Model file for the job. Use its own axes, mm. A direction names the side the tool comes from. Round coordinates to 2 decimals unless told otherwise and drop trailing zeros. Order: outer loops, then holes, each group sorted by start corner. A loop starts at its lowest first (then second) coordinate and runs counter-clockwise, first axis right, second up. Notation, with made-up numbers: (23.5, -34.75) - (65.5, -34.75) arc R16 ccw to (65.5, -13.75) - close; hole circle Ø5 at (33.5, 88.25). An arc over 180 degrees is marked (long way). Put each result on its own line as item: value. Start each with the question number.
Item 1: Saw through at B-B on x = 11. List the corners of the cut face in (y, z).
Item 2: Probe probe 1 along Z at (x, y) = (5.5, 0); probe 2 along Z at (x, y) = (3.5, 0); probe 3 along Y at (x, z) = (5, 1.5). List the from-to ranges inside material, lowest first.
Item 3: Pin check, flat tips, straight feed: pin 1 Ø5 at (x, z) = (17, 2) entering from -Y; pin 2 Ø3 at (y, z) = (0, 0) entering from -X; pin 3 Ø3 at (x, y) = (11.5, -4.5) entering from +Z. Stop position of each tip, or through.
Item 4: Saw through at A-A on x = 5.5. List the corners of the cut face in (y, z).
Item 5: Which spindle directions (+Z, -Z, +X, -X, +Y, -Y) get a long thin tool onto all of the face, cutting with end or side? Do faces 1 (the face through (4, 0, -2)), 2 (the face through (28.578, -2, 5)). Say none if no direction does.
Item 6: Mould opens along Z. For faces 3 (the face through (2.028, -0.867, -3.905)), 4 (the face through (19.56, -2.05, -1.57)), 5 (the face through (4, 4.3, 0.1)) say: pulls with the +Z half, pulls with the -Z half, needs draft (parallel to the pull), parting line crosses it, or undercut.
Autodesk Inventor part; units mm, degrees
ref_plane "YZ Plane" through (0, 0, 0) normal (1, 0, 0) x (0, 1, 0)
ref_plane "XZ Plane" through (0, 0, 0) normal (0, 1, 0) x (-1, 0, 0)
ref_plane "XY Plane" through (0, 0, 0) normal (0, 0, 1) x (1, 0, 0)
sketch "Sketch1" plane through (0, 0, 0) normal (0, 0, 1) x (1, 0, 0)
  line L0 (0, 0) -> (0, 2)
  line L1 (0, 2) -> (50, 2)
  line L2 (0, 0) -> (0, 0.1)
  line L3 (0, 0.1) -> (50, 0.1)
  line L4 (0, 0) -> (0, 5)
  line L5 (0, 5) -> (50, 5)
  line L6 (0, 0) -> (0, 4)
  line L7 (0, 4) -> (4, 4)
  line L8 (4, 4) -> (4, 2)
  line L9 (4, 2) -> (4, 10)
  line L10 (4, 2) -> (6.7109, 2) construction
  line L11 (4, 10) -> (7, 10)
  line L12 (7, 10) -> (7, 2)
  line L13 (7, 2) -> (10.2909, 0.1)
  line L14 (7, 2) -> (9.25, 2) construction
  line L15 (10.2909, 0.1) -> (28.5779, 5)
  line L16 (10.2909, 0.1) -> (29.223, 0.1) construction
  line L17 (28.5779, 5) -> (28.5779, 7)
  line L18 (28.5779, 7) -> (7, 10)
  line L19 (0, 0) -> (50, 0)
  line L20 (-10, 0) -> (60, 0)
  point P0 (0, 2)
  point P1 (7, 5)
  point P2 (4, 5)
  point P3 (17.0086, 2)
  point P4 (17.3818, 2)
  dimension "d0" = 2
  dimension "d1" = 50
  dimension "d2" = 0.1
  dimension "d3" = 5
  dimension "d4" = 4
  dimension "d5" = 4
  dimension "d6" = 8
  dimension "d8" = 3
  dimension "d9" = 30
  dimension "d10" = 15
  dimension "d13" = 50
revolve "Revolution2" add sketch "Sketch1" angle 360 about axis through (-10, 0, 0) along (1, 0, 0) contours L4 L7 L8 L1 | L13 L1 L15 | L8 L9 L5 L12 L1 | L12 L5 L15 L1 | L12 L18 L17 L5 | L5 L9 L11 L12
thread "Thread3"
Results found:
1. outline: circle Ø18.89 at (0, 0); hole circle Ø0.58 at (0, 0)
2. probe 1: z = -10 to -2, 2 to 10
2. probe 2: z = -4 to -2, 2 to 4
2. probe 3: y = -9.89 to -1.32, 1.32 to 9.89
3. pin 1: stops at y = -8.88
3. pin 2: stops at x = 7.87
3. pin 3: stops at z = 8.93
4. outline: circle Ø20 at (0, 0); hole circle Ø4 at (0, 0)
5. face 1: -X
5. face 2: +Z, -Z, +X, +Y, -Y
6. face 3: parting line crosses it
6. face 4: undercut
6. face 5: needs draft
